Part model, mm, in its own coordinate system. A direction names the side the tool comes from. Round coordinates to 2 decimals unless told otherwise and drop trailing zeros. Loops run counter-clockwise (first coordinate to the right, second up) from the corner with the lowest first, then second, coordinate; pieces in that order, holes last.
1) Band-saw the part on D-D, the plane z = 12. Write the cut outline in (x, y).
2) Band-saw the part on C-C, the plane y = -2.5. State how many separate pieces and enclosed holes the cut face has, then the cut area to 3 significant figures.
3) 3-axis set-ups, long thin cutter, end or side, ignore diameter. For faces 5 (the flat face through (6, -7.62, 11)), 6 (the conical face through (-0.03, -1.41, 14.87)): which of +Z, -Z, +X, -X, +Y, -Y reach the whole face in a straight line?
4) Probe line 1 (Z direction, x = -5.5, y = -6); line 2 (X direction, y = -3.75, z = 4.5); line 3 (Z direction, x = 5.25, y = -5.25). List the from-to ranges inside material, lowest first.
5) Band-saw the part on B-B, the plane z = 3.5. Write the cut outline in (x, y).
6) Drop flat-ended pins along their axis: P1, Ø2, axis at x = 9, z = 6.5, coming from the -Y side; P2, Ø1.2, axis at x = 6.5, z = 10, coming from the +Y side; P3, Ø5, axis at x = -6.096, z = 4.191, coming from the -Y side. Give the stop position or say it passes through.
7) Mould opens along X. For faces 1 (the conical face through (-0.031, -1.414, 0.363)), 2 (the flat face through (6, 0, 8)), 3 (the flat face through (-6, -7.62, 11)), 4 (the cylindrical face through (0.251, -11.427, 7.52)) say: +X half, -X half, draft (parallel to the pull), parting line (faces both ways), or undercut.
8) Band-saw the part on A-A, the plane x = 0. Write the cut outline in (y, z), then the cut area to 3 significant figures.
from build123d import *

# Parameters (mm, degrees)
BOSS_EXTRUDE2_DEPTH = 15.24
CHAMFER1_SIZE       = 0.508
CHAMFER2_SIZE       = 0.508
SKETCH13_R          = 1.9558
CUT_EXTRUDE1_DEPTH  = 7.62


with BuildPart() as part:
    # Sketch9 → Boss-Extrude2 (new body)
    with BuildSketch(Plane.XY):
        with BuildLine():
            Line((-11.43, 0), (-1.27, 0))
            ThreePointArc((-1.27, 0), (0, -1.27), (1.27, 0))
            Line((1.27, 0), (11.43, 0))
            ThreePointArc((11.43, 0), (0, -11.43), (-11.43, 0))
        make_face()
    extrude(amount=BOSS_EXTRUDE2_DEPTH)

    # Chamfer1
    chamfer1_edges = [part.edges().sort_by_distance(p)[0] for p in [
        (6.35, 0, 0),
        (0, -11.43, 0),
        (-6.35, 0, 0),
        (0, -1.27, 0),
    ]]
    chamfer(chamfer1_edges, length=CHAMFER1_SIZE)

    # Chamfer2
    chamfer2_edges = [part.edges().sort_by_distance(p)[0] for p in [
        (0, -11.43, 15.24),
        (6.35, 0, 15.24),
        (0, -1.27, 15.24),
        (-6.35, 0, 15.24),
    ]]
    chamfer(chamfer2_edges, length=CHAMFER2_SIZE)

    # Sketch13 → Cut-Extrude1 (cut)
    with BuildSketch(Plane(origin=(0, 0, 0), x_dir=(1, 0, 0), z_dir=(0, 1, 0))):
        with Locations((-6.096, -4.191)):
            Circle(SKETCH13_R)
        with Locations((-6.096, -11.049)):
            Circle(SKETCH13_R)
        with Locations((6.096, -11.049)):
            Circle(SKETCH13_R)
        with Locations((6.096, -4.191)):
            Circle(SKETCH13_R)
    extrude(amount=-CUT_EXTRUDE1_DEPTH, mode=Mode.SUBTRACT)


solid = part.part
Reported:
1. outline: (-11.43, 0) arc R11.43 ccw to (11.43, 0) - (7.81, 0) - (7.81, -7.62) - (4.39, -7.62) - (4.39, 0) - (1.27, 0) arc R1.27 cw to (-1.27, 0) - (-4.39, 0) - (-4.39, -7.62) - (-7.81, -7.62) - (-7.81, 0) - close
2. separate pieces: 1
2. enclosed holes: 4
2. area: 291 mm2
3. face 5: +Y
3. face 6: +Z, +Y
4. line 1: z = 0 to 2.33, 6.05 to 9.19, 12.91 to 15.24
4. line 2: x = -10.8 to -8.03, -4.16 to 4.16, 8.03 to 10.8
4. line 3: z = 0 to 2.43, 5.95 to 9.29, 12.81 to 15.24
5. outline: (-11.43, 0) arc R11.43 ccw to (11.43, 0) - (7.93, 0) - (7.93, -7.62) - (4.27, -7.62) - (4.27, 0) - (1.27, 0) arc R1.27 cw to (-1.27, 0) - (-4.27, 0) - (-4.27, -7.62) - (-7.93, -7.62) - (-7.93, 0) - close
6. P1: stops at y = -8.16
6. P2: stops at y = -7.62
6. P3: stops at y = -10.85
7. face 1: undercut
7. face 2: draft
7. face 3: undercut
7. face 4: parting line
8. outline: (-11.43, 0.51) - (-10.92, 0) - (-1.78, 0) - (-1.27, 0.51) - (-1.27, 14.73) - (-1.78, 15.24) - (-10.92, 15.24) - (-11.43, 14.73) - close
8. area: 154 mm2
